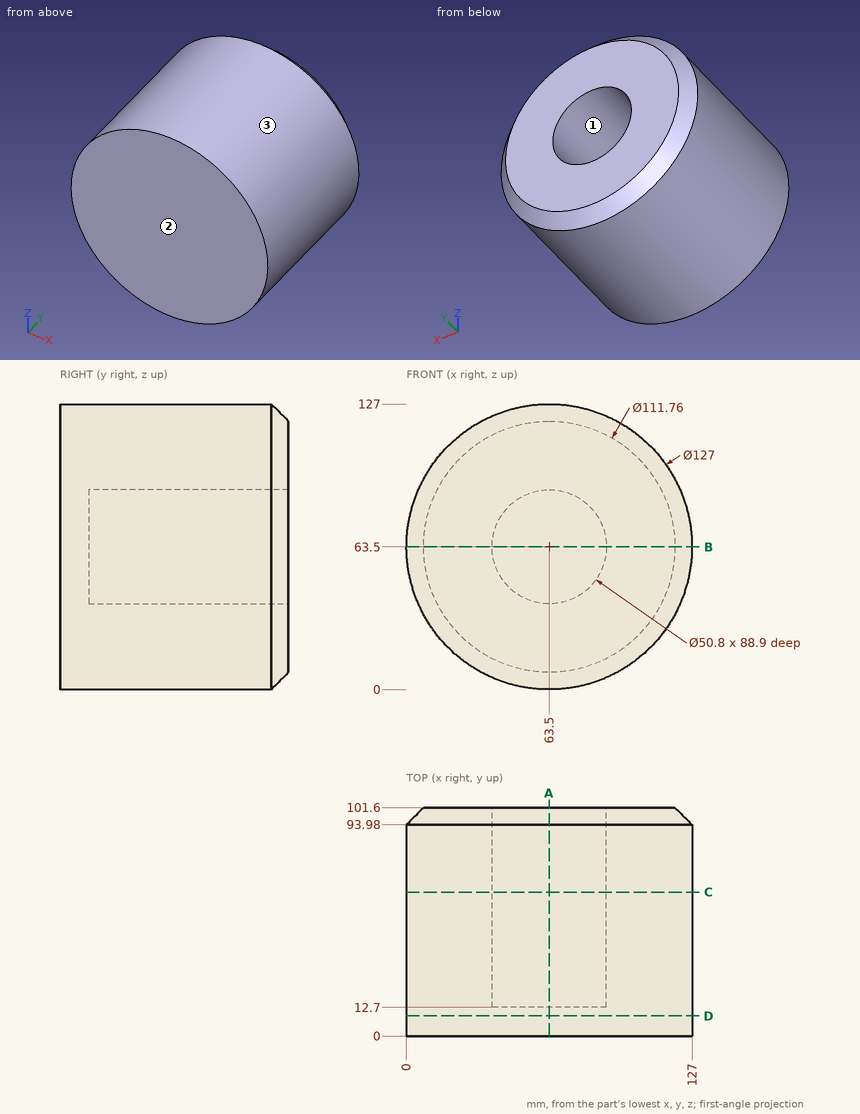
Input: dimensioned drawing with shaded views. Units: mm. Origin: part minimum x, y, z. Give positions to 0.01 mm unless a question says otherwise; leave off trailing zeros. Write each loop counter-clockwise with the first axis right and the second up, starting at its lowest first coordinate (ties: lowest second). Pieces come first, ordered by that corner, then holes.
Q1. Section B-B, the plane z = 63.5. Output: boundary loops of the cut face in (x, y).
Q2. First-contact query: P1, Ø1, axis at y = 32, z = 65.5, coming from the -X side; P2, Ø3, axis at x = 71, z = 87, coming from the +Y side; P3, Ø8, axis at y = 63, z = 28, coming from the -X side; P4, Ø4, axis at x = 46.5, y = 55, coming from the +Z side. Flat tips, straight axial feed; report the tip coordinate or a pass-through.
Q3. Material intervals for probe 1 along X at (y, z) = (69, 63.5); probe 2 along Y at (x, z) = (58.5, 41), sorted ascending.
Q4. Section D-D, the plane y = 9. Output: boundary loops of the cut face in (x, z).
Q5. Section C-C, the plane y = 64. Output: boundary loops of the cut face in (x, z).
Q6. Pull-direction query (X, two-part tool) for the marked faces 1, 2 and 3; classes: pulls with the +X half, pulls with the -X half, needs draft (parallel to the pull), parting line crosses it, or undercut.
Q7. Section A-A, the plane x = 63.5. Output: boundary loops of the cut face in (y, z).
Filled in:
1. outline: (0, 0) - (127, 0) - (127, 93.98) - (119.38, 101.6) - (88.9, 101.6) - (88.9, 12.7) - (38.1, 12.7) - (38.1, 101.6) - (7.62, 101.6) - (0, 93.98) - close
2. P1: stops at x = 0.02
2. P2: stops at y = 101.6
2. P3: stops at x = 8.36
2. P4: stops at z = 125.2
3. probe 1: x = 0 to 38.1, 88.9 to 127
3. probe 2: y = 0 to 12.7
4. outline: circle Ø127 at (63.5, 63.5)
5. outline: circle Ø127 at (63.5, 63.5); hole circle Ø50.8 at (63.5, 63.5)
6. face 1: undercut
6. face 2: needs draft
6. face 3: parting line crosses it
7. outline: (0, 0) - (93.98, 0) - (101.6, 7.62) - (101.6, 38.1) - (12.7, 38.1) - (12.7, 88.9) - (101.6, 88.9) - (101.6, 119.38) - (93.98, 127) - (0, 127) - close
